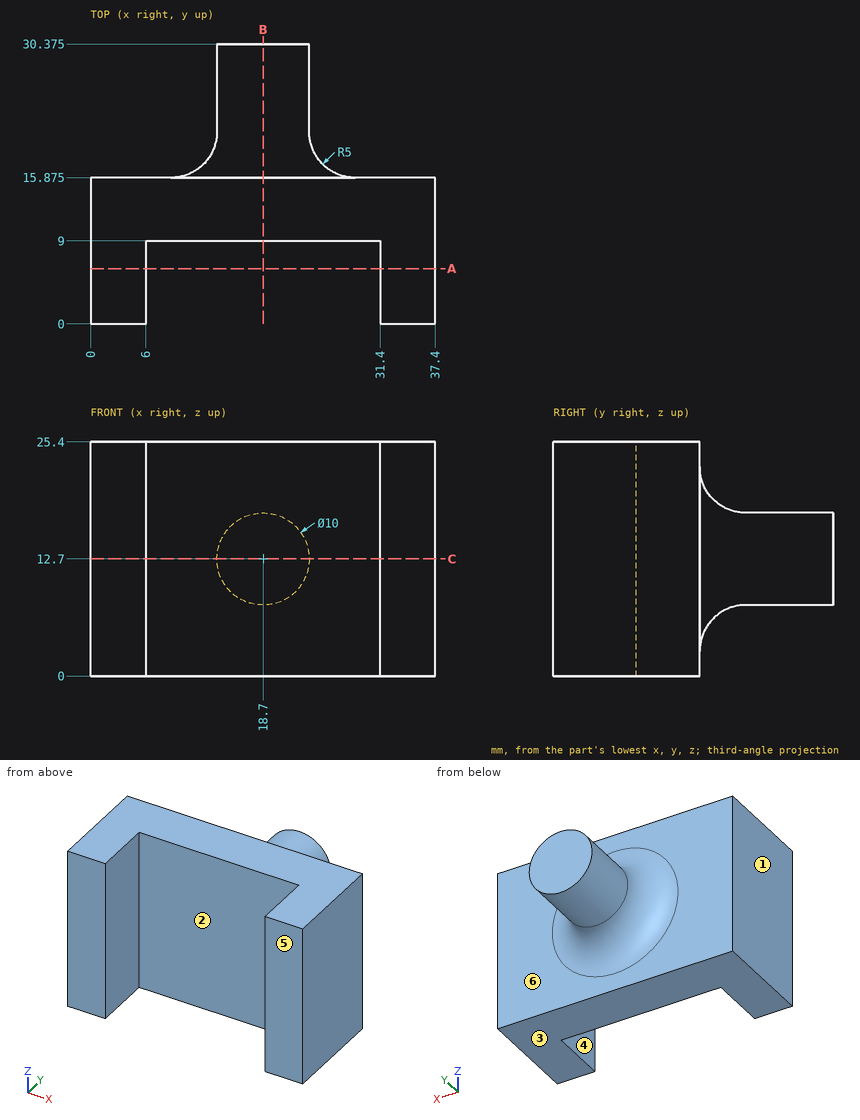
The drawing under review shows one solid part. Ordinate dimensions are in mm from its lowest x, y, z. A direction names the side the tool comes from. Coordinates: 2 decimals unless noted, no trailing zeros. Order: outer loops, then holes, each group sorted by start corner. A loop starts at its lowest first (then second) coordinate and runs counter-clockwise, first axis right, second up. Notation, with made-up numbers: (64, 21.5) -> (95, 21.5) arc R23 ccw to (95, 44.5) -> close; hole circle Ø2 at (66, 54.5). An arc over 180 degrees is marked (long way). One line per item, written item: value.
1) We need section A-A, the plane y = 6. Give the boundary of the cut face in (x, z).
Output values:
outline: (0, 0) -> (6, 0) -> (6, 25.4) -> (0, 25.4) -> close; (31.4, 0) -> (37.4, 0) -> (37.4, 25.4) -> (31.4, 25.4) -> close
2) Machinability: for the marked faces 4, 5 and 6, which of the approach directions +Z, -Z, +X, -X, +Y, -Y give a long, thin tool a straight path to every point of the face, cutting with its end or side? Answer none if there is none.
Output values:
face 4: +Z, -Z, -Y
face 5: +Z, -Z, +X, -X, -Y
face 6: +Y
3) We need section B-B, the plane x = 18.7. Give the boundary of the cut face in (y, z) (3 decimals), then the cut area to 3 significant figures.
Output values:
outline: (9, 0) -> (15.875, 0) -> (15.875, 2.7) arc R5 cw to (20.875, 7.7) -> (30.375, 7.7) -> (30.375, 17.7) -> (20.875, 17.7) arc R5 cw to (15.875, 22.7) -> (15.875, 25.4) -> (9, 25.4) -> close
area: 330 mm2
4) To check wall thickness, follow probe 1 along X at (y, z) = (7, 5); probe 2 along Y at (x, z) = (28, 2.5) (3 decimals); probe 3 along Y at (x, z) = (14, 14) (3 decimals). State the ranges of each line that lie inside material, in increasing order. Write a range as [from, to].
Output values:
probe 1: x = [0, 6], [31.4, 37.4]
probe 2: y = [9, 15.875]
probe 3: y = [9, 30.375]
5) Clearance check with flat-ended pins moving along their axes: P1, Ø3, axis at x = 20, z = 11, coming from the -Y side; P2, Ø3, axis at x = 8.5, z = 15, coming from the +Y side; P3, Ø1, axis at x = 23, y = 17, coming from the -Z side. State where each tip first meets the part, or that it passes through.
Output values:
P1: stops at y = 9
P2: stops at y = 15.99
P3: stops at z = 6.41
6) Draft analysis for pull direction X (two halves, no side actions). For the marked faces 1, 2 and 3, state which applies: +X half, -X half, draft (parallel to the pull), parting line (faces both ways), or undercut.
Output values:
face 1: -X half
face 2: undercut
face 3: draft
7) We need section C-C, the plane z = 12.7. Give the boundary of the cut face in (x, y) (3 decimals), then the cut area to 3 significant figures.
Output values:
outline: (0, 0) -> (6, 0) -> (6, 9) -> (31.4, 9) -> (31.4, 0) -> (37.4, 0) -> (37.4, 15.875) -> (28.7, 15.875) arc R5 cw to (23.7, 20.875) -> (23.7, 30.375) -> (13.7, 30.375) -> (13.7, 20.875) arc R5 cw to (8.7, 15.875) -> (0, 15.875) -> close
area: 521 mm2
